```python
from build123d import *

# Parameters (mm, degrees)
SKETCH_1_R          = 1.65
EXTRUDE_1_DEPTH     = 3
CUT_EXTRUDE_1_DEPTH = 172.458449777


with BuildPart() as part:
    # 草图1 → 凸台-拉伸1 (new body)
    with BuildSketch(Plane(origin=(0, 0, 0), x_dir=(1, 0, 0), z_dir=(0, 1, 0))):
        Polygon((0, 0), (13, 0), (13, -3), (25, -3), (25, 0), (125, 0), (125, -3), (137, -3), (137, 0), (150, 0), (150, 80), (137, 80), (137, 83), (125, 83), (125, 80), (25, 80), (25, 83), (13, 83), (13, 80), (0, 80), align=None)
        with Locations(Location((35, 73.8, 0), (0, 0, 270))):
            Circle(SKETCH_1_R, mode=Mode.SUBTRACT)
        with Locations(Location((35, 46.2, 0), (0, 0, 270))):
            Circle(SKETCH_1_R, mode=Mode.SUBTRACT)
        with Locations(Location((115, 46.2, 0), (0, 0, 90))):
            Circle(SKETCH_1_R, mode=Mode.SUBTRACT)
        with Locations(Location((115, 73.8, 0), (0, 0, 90))):
            Circle(SKETCH_1_R, mode=Mode.SUBTRACT)
        with Locations(Location((35, 36.2, 0), (0, 0, 90))):
            Circle(SKETCH_1_R, mode=Mode.SUBTRACT)
        with Locations(Location((70, 46.2, 0), (0, 0, 90))):
            Circle(SKETCH_1_R, mode=Mode.SUBTRACT)
        with Locations(Location((70, 36.2, 0), (0, 0, 90))):
            Circle(SKETCH_1_R, mode=Mode.SUBTRACT)
        with BuildLine():
            Line((13, 42.4), (25, 42.4))
            ThreePointArc((25, 42.4), (26.7, 40.7), (25, 39))
            Line((25, 39), (13, 39))
            ThreePointArc((13, 39), (11.3, 40.7), (13, 42.4))
        make_face(mode=Mode.SUBTRACT)
        with BuildLine():
            Line((125, 42.4), (137, 42.4))
            ThreePointArc((137, 42.4), (138.7, 40.7), (137, 39))
            Line((137, 39), (125, 39))
            ThreePointArc((125, 39), (123.3, 40.7), (125, 42.4))
        make_face(mode=Mode.SUBTRACT)
    extrude(amount=EXTRUDE_1_DEPTH)

    # 草图2 → 切除-拉伸1 (cut, through all)
    with BuildSketch(Plane(origin=(0, 3, 0), x_dir=(1, 0, 0), z_dir=(0, 1, 0))):
        Polygon((43.3, 0), (43.3, 3.5), (42, 3.5), (42, 7), (43.3, 7), (43.3, 10.4), (46.7, 10.4), (46.7, 7), (48, 7), (48, 3.5), (46.7, 3.5), (46.7, 0), align=None)
        Polygon((103.3, 0), (106.7, 0), (106.7, 3.5), (108, 3.5), (108, 7), (106.7, 7), (106.7, 10.4), (103.3, 10.4), (103.3, 7), (102, 7), (102, 3.5), (103.3, 3.5), align=None)
    extrude(amount=-CUT_EXTRUDE_1_DEPTH, mode=Mode.SUBTRACT)


solid = part.part
```
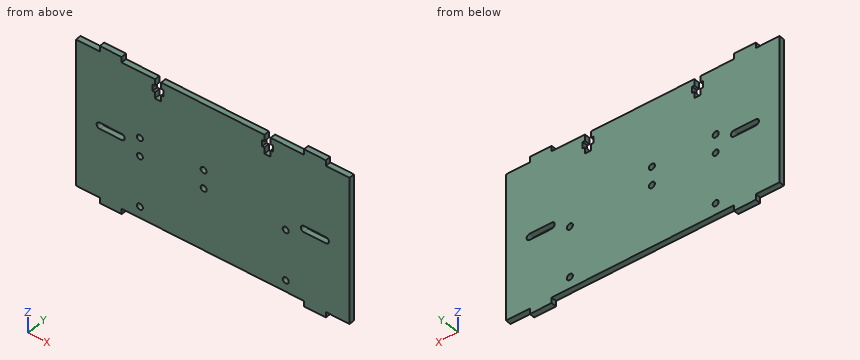
Read the model definition and answer for the solid it produces. Units are mm, in the model's axes. Round coordinates to 2 decimals unless told otherwise and drop trailing zeros. Write each loop counter-clockwise with the first axis right and the second up, starting at its lowest first coordinate (ties: lowest second). Pieces come first, ordered by that corner, then holes. Notation, with made-up numbers: (3, 39) - (34, 39) arc R27 ccw to (34, 74) - close; hole circle Ø4 at (45, -2). An arc over 180 degrees is marked (long way). Use CSV: the item, a comma, the result in double quotes.
Q1. Straight lines are drawn through the part: line 1 along X through (y, z) = (1.9, -36.2); line 2 along Z through (x, y) = (70, 1.1); line 3 along X through (y, z) = (0.7, -46.2). For each, find the intervals that lie inside material, in ascending order.
Values:
line 1,"x = 0 to 33.35, 36.65 to 68.35, 71.65 to 150"
line 2,"z = -80 to -47.85, -44.55 to -37.85, -34.55 to 0"
line 3,"x = 0 to 33.35, 36.65 to 68.35, 71.65 to 113.35, 116.65 to 150"
Q2. Find section A-A, the plane z = -46.2. Write down the section's boundary in (x, y), then the cut area to 3 significant figures.
Values:
outline,"(0, 0) - (33.35, 0) - (33.35, 3) - (0, 3) - close; (36.65, 0) - (68.35, 0) - (68.35, 3) - (36.65, 3) - close; (71.65, 0) - (113.35, 0) - (113.35, 3) - (71.65, 3) - close; (116.65, 0) - (150, 0) - (150, 3) - (116.65, 3) - close"
area,"420 mm²"
Q3. Find section B-B, the plane x = 129. Write down the section's boundary in (y, z), then the cut area to 3 significant figures.
Values:
outline,"(0, -83) - (3, -83) - (3, -42.4) - (0, -42.4) - close; (0, -39) - (3, -39) - (3, 3) - (0, 3) - close"
area,"248 mm²"
Q4. Find section C-C, the plane z = -73.8. Write down the section's boundary in (x, y).
Values:
outline,"(0, 0) - (33.35, 0) - (33.35, 3) - (0, 3) - close; (36.65, 0) - (113.35, 0) - (113.35, 3) - (36.65, 3) - close; (116.65, 0) - (150, 0) - (150, 3) - (116.65, 3) - close"
Q5. Find section D-D, the plane y = 1.2. Count the separate pieces of the cut face and the enclosed holes in it, then the cut area to 3 significant figures.
Values:
separate pieces,"1"
enclosed holes,"9"
area,"11,900 mm²"
Q6. Each of these flat-tipped pins is pushed along its axis until it touches: pin 1 Ø5.5 at (x, z) = (70, -36.2) entering from -Y; pin 2 Ø1 at (x, y) = (109, 2.5) entering from -Z; pin 3 Ø3 at (x, z) = (35, -73.8) entering from -Y; pin 4 Ø0.6 at (x, y) = (47.5, 1) entering from +Z. Where does it stop, or does it pass through?
Values:
pin 1,"stops at y = 0"
pin 2,"stops at z = -80"
pin 3,"passes through"
pin 4,"stops at z = 0"
